```python
from build123d import *

# Parameters (mm, degrees)
SKETCH_2_W          = 80
SKETCH_2_H          = 140
EXTRUDE_1_DEPTH     = 4
SKETCH_3_R          = 1.8
SKETCH_3_R_2        = 2.35
SKETCH_3_R_3        = 2.5
CUT_EXTRUDE_3_DEPTH = 4


with BuildPart() as part:
    # 草图2 → 凸台-拉伸1 (new body)
    with BuildSketch(Plane(origin=(0, 0, 0), x_dir=(1, 0, 0), z_dir=(0, 1, 0))):
        with Locations((-40, 0)):
            Rectangle(SKETCH_2_W, SKETCH_2_H)
    extrude(amount=EXTRUDE_1_DEPTH)

    # 草图3 → 切除-拉伸3 (cut)
    with BuildSketch(Plane(origin=(0, 4, 0), x_dir=(1, 0, 0), z_dir=(0, 1, 0))):
        with Locations(Location((-72, 63.5, 0), (0, 0, 270))):
            Circle(SKETCH_3_R)
        with Locations(Location((-41, 63.5, 0), (0, 0, 270))):
            Circle(SKETCH_3_R)
        with Locations(Location((-41, 36.5, 0), (0, 0, 270))):
            Circle(SKETCH_3_R)
        with Locations(Location((-72, 36.5, 0), (0, 0, 270))):
            Circle(SKETCH_3_R)
        with Locations(Location((-41, -63.5, 0), (0, 0, 270))):
            Circle(SKETCH_3_R)
        with Locations(Location((-41, -36.5, 0), (0, 0, 270))):
            Circle(SKETCH_3_R)
        with Locations(Location((-72, -36.5, 0), (0, 0, 270))):
            Circle(SKETCH_3_R)
        with Locations(Location((-72, -63.5, 0), (0, 0, 270))):
            Circle(SKETCH_3_R)
        with Locations(Location((-73.9, 50, 0), (0, 0, 270))):
            Circle(SKETCH_3_R_2)
        with Locations(Location((-73.9, -50, 0), (0, 0, 270))):
            Circle(SKETCH_3_R_2)
        with Locations(Location((-39.1, -50, 0), (0, 0, 270))):
            Circle(SKETCH_3_R_2)
        with Locations(Location((-39.1, 50, 0), (0, 0, 270))):
            Circle(SKETCH_3_R_2)
        with Locations(Location((-10, 60, 0), (0, 0, 270))):
            Circle(SKETCH_3_R_3)
        with Locations(Location((-10, 0, 0), (0, 0, 270))):
            Circle(SKETCH_3_R_3)
        with Locations(Location((-10, -60, 0), (0, 0, 270))):
            Circle(SKETCH_3_R_3)
    extrude(amount=-CUT_EXTRUDE_3_DEPTH, mode=Mode.SUBTRACT)


solid = part.part
```
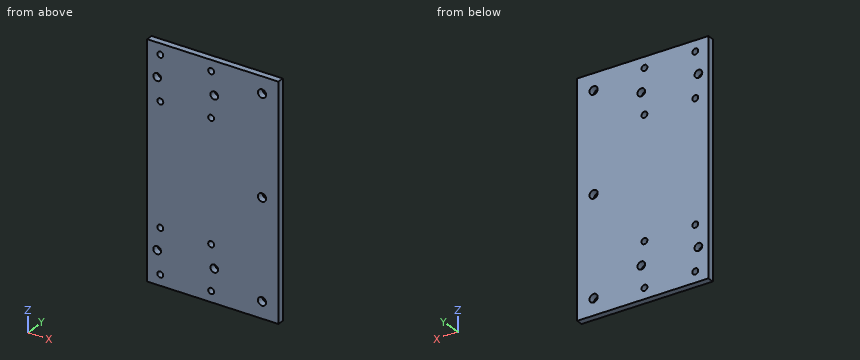
Source: CAD feature listing. Evaluate the final solid. Frame: model axes, mm. Coordinates: 2 decimals unless noted, no trailing zeros. Order: outer loops, then holes, each group sorted by start corner. A loop starts at its lowest first (then second) coordinate and runs counter-clockwise, first axis right, second up. Notation, with made-up numbers: M 26.25,56.5 L 50.25,56.5 A26 ccw 50.25,95.5 Z; hole C 82.5,-20 d5. An arc over 180 degrees is marked long. Write each question's results on one line, items separated by ' | '. Start each with the question number.
1) Line query: line 1 (X direction, y = 2.3, z = -36.5); line 2 (X direction, y = 3, z = -50); line 3 (Z direction, x = -71, y = 3). Output: solid intervals per line, ascending. Write a range as from..to.
2) Section query C-C (z = 0). Return the cut outline in (x, y).
3) Section query B-B (x = -10). Return the cut outline in (y, z), plus the area to 3 significant figures.
4) Contact query for a flat-ended pin moving along its axis: pin 1 Ø3 at (x, z) = (-41, 36.5) entering from +Y. Output: stop coordinate, or through.
5) Section query D-D (y = 1.3). Give the number of separate pieces and of enclosed holes in the cut face, plus the area to 3 significant figures.
6) Section query A-A (z = 36.5). Return the cut outline in (x, y).
Answers:
1) line 1: x = -80..-73.8, -70.2..-42.8, -39.2..0 | line 2: x = -80..-76.25, -71.55..-41.45, -36.75..0 | line 3: z = -70..-65, -62..-38, -35..35, 38..62, 65..70
2) outline: M -80,0 L -12.5,0 L -12.5,4 L -80,4 Z; M -7.5,0 L 0,0 L 0,4 L -7.5,4 Z
3) outline: M 0,-70 L 4,-70 L 4,-62.5 L 0,-62.5 Z; M 0,-57.5 L 4,-57.5 L 4,-2.5 L 0,-2.5 Z; M 0,2.5 L 4,2.5 L 4,57.5 L 0,57.5 Z; M 0,62.5 L 4,62.5 L 4,70 L 0,70 Z | area: 500 mm^2
4) pin 1: passes through
5) separate pieces: 1 | enclosed holes: 15 | area: 11,000 mm^2
6) outline: M -80,0 L -73.8,0 L -73.8,4 L -80,4 Z; M -70.2,0 L -42.8,0 L -42.8,4 L -70.2,4 Z; M -39.2,0 L 0,0 L 0,4 L -39.2,4 Z
